For this review, take the finished solid that the model builds, in its own axes (mm). Face numbers are marked on the shaded views. A direction names the side the tool comes from. Give positions to 0.01 mm unless a question says otherwise; leave off trailing zeros. Write each loop counter-clockwise with the first axis right and the second up, starting at its lowest first coordinate (ties: lowest second). Pieces come first, ordered by that corner, then holes. Notation, with made-up numbers: (9.5, 15.25) -> (19.5, 15.25) arc R30 cw to (19.5, 40.25) -> close; hole circle Ø7 at (25.5, 88.25). An arc over 180 degrees is marked (long way). Return JSON: item names as keys, results as strings.
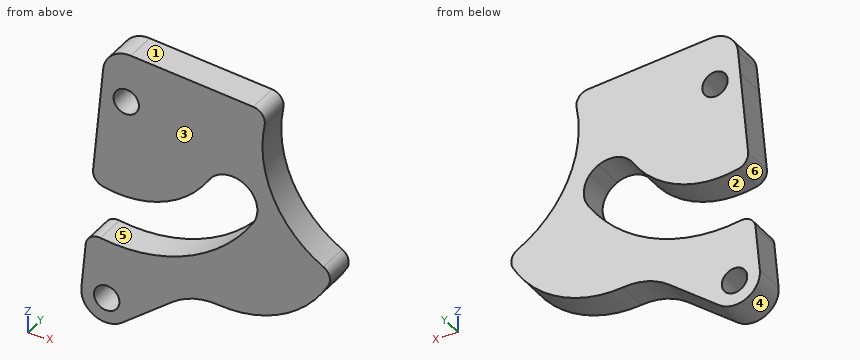
from build123d import *

# Parameters (mm, degrees)
SKETCH_1_R          = 2
EXTRUDE_1_DEPTH     = 5
EXTRUDE_2_DEPTH     = 5
CUT_EXTRUDE_1_DEPTH = 6
EXTRUDE_3_DEPTH     = 5
FILLET_1_R          = 10
FILLET_2_R          = 2
SKETCH_6_R          = 18.75
CUT_EXTRUDE_2_DEPTH = 6
FILLET_3_R          = 2


with BuildPart() as part:
    # 草图1 → 凸台-拉伸1 (new body)
    with BuildSketch(Plane(origin=(0, 0, 0), x_dir=(1, 0, 0), z_dir=(0, 1, 0))):
        with BuildLine():
            ThreePointArc((-20.0875, 4), (-23.044826598, 2.693365811), (-24.070081176, -0.372890305))
            ThreePointArc((-24.070081176, -0.372890305), (-22.780865811, -2.957326598), (-20.0875, -4))
            ThreePointArc((-20.0875, -4), (-17.130173402, -2.693365811), (-16.104918824, 0.372890305))
            Line((-16.104918824, 0.372890305), (-16.444526225, 4))
            Line((-16.444526225, 4), (-20.0875, 4))
        make_face()
        with Locations((-20.0875, 0)):
            Circle(SKETCH_1_R, mode=Mode.SUBTRACT)
        with BuildLine():
            Line((-27.14754486, 32.495352138), (-24.070081176, -0.372890305))
            ThreePointArc((-24.070081176, -0.372890305), (-23.044826598, 2.693365811), (-20.0875, 4))
            Line((-20.0875, 4), (-16.444526225, 4))
            Line((-16.444526225, 4), (-18.333300994, 24.172685504))
            Line((-18.333300994, 24.172685504), (-25.585127327, 29.683464909))
            ThreePointArc((-25.585127327, 29.683464909), (-26.661456606, 30.925425609), (-27.14754486, 32.495352138))
        make_face()
        with BuildLine():
            ThreePointArc((-20.74480004, 36.053019976), (-25.107780517, 36.364735365), (-27.14754486, 32.495352138))
            ThreePointArc((-27.14754486, 32.495352138), (-26.661456606, 30.925425609), (-25.585127327, 29.683464909))
            Line((-25.585127327, 29.683464909), (-18.333300994, 24.172685504))
            Line((-18.333300994, 24.172685504), (-19.182382508, 33.241132747))
            ThreePointArc((-19.182382508, 33.241132747), (-19.668470762, 34.811059276), (-20.74480004, 36.053019976))
        make_face()
        with Locations((-23.164963684, 32.868242443)):
            Circle(SKETCH_1_R, mode=Mode.SUBTRACT)
        with BuildLine():
            Line((22.507663644, 3.184777534), (-20.74480004, 36.053019976))
            ThreePointArc((-20.74480004, 36.053019976), (-19.668470762, 34.811059276), (-19.182382508, 33.241132747))
            Line((-19.182382508, 33.241132747), (-18.333300994, 24.172685504))
            Line((-18.333300994, 24.172685504), (8.212637649, 4))
            Line((8.212637649, 4), (20.0875, 4))
            ThreePointArc((20.0875, 4), (21.364388771, 3.790719598), (22.507663644, 3.184777534))
        make_face()
        with BuildLine():
            ThreePointArc((-16.104918824, 0.372890305), (-17.130173402, -2.693365811), (-20.0875, -4))
            Line((-20.0875, -4), (20.0875, -4))
            ThreePointArc((20.0875, -4), (18.810611229, -3.790719598), (17.667336356, -3.184777534))
            Line((17.667336356, -3.184777534), (8.212637649, 4))
            Line((8.212637649, 4), (-16.444526225, 4))
            Line((-16.444526225, 4), (-16.104918824, 0.372890305))
        make_face()
        with BuildLine():
            ThreePointArc((17.667336356, -3.184777534), (18.810611229, -3.790719598), (20.0875, -4))
            ThreePointArc((20.0875, -4), (23.878219598, -1.276888771), (22.507663644, 3.184777534))
            ThreePointArc((22.507663644, 3.184777534), (21.364388771, 3.790719598), (20.0875, 4))
            Line((20.0875, 4), (8.212637649, 4))
            Line((8.212637649, 4), (17.667336356, -3.184777534))
        make_face()
        with Locations((20.0875, 0)):
            Circle(SKETCH_1_R, mode=Mode.SUBTRACT)
        Polygon((-18.333300994, 24.172685504), (-16.444526225, 4), (8.212637649, 4), align=None)
    extrude(amount=EXTRUDE_1_DEPTH)

    # 草图2 → 凸台-拉伸2 (add)
    with BuildSketch(Plane(origin=(0, 5, 0), x_dir=(1, 0, 0), z_dir=(0, 1, 0))):
        with BuildLine():
            ThreePointArc((-20.0875, -4), (-22.780865811, -2.957326598), (-24.070081176, -0.372890305))
            Line((-24.070081176, -0.372890305), (-23.720962628, -4.10158193))
            ThreePointArc((-23.720962628, -4.10158193), (-22.290826699, -6.808468121), (-19.365512753, -7.711274824))
            Line((-19.365512753, -7.711274824), (20.460368699, -3.982583199))
            ThreePointArc((20.460368699, -3.982583199), (20.274137625, -3.995643427), (20.0875, -4))
            Line((20.0875, -4), (-20.0875, -4))
        make_face()
    extrude(amount=-EXTRUDE_2_DEPTH)

    # 草图3 → 切除-拉伸1 (cut, through all)
    with BuildSketch(Plane(origin=(0, 5, 0), x_dir=(1, 0, 0), z_dir=(0, 1, 0))):
        with BuildLine():
            ThreePointArc((-36.289327432, 17.433897667), (-37.629570165, 14.285674695), (-36.182704661, 11.185007239))
            ThreePointArc((-36.182704661, 11.185007239), (-31.653466249, 15.823666602), (-25.858788976, 18.731049718))
            Line((-25.858788976, 18.731049718), (-26.257218708, 22.986399698))
            ThreePointArc((-26.257218708, 22.986399698), (-31.612650276, 20.82332613), (-36.289327432, 17.433897667))
        make_face()
        with BuildLine():
            ThreePointArc((-25.858788976, 18.731049718), (-11.47348363, 17.605644606), (-1.756724615, 6.938492183))
            ThreePointArc((-1.756724615, 6.938492183), (0.40025314, 9.594618202), (-0.134776474, 12.974159854))
            ThreePointArc((-0.134776474, 12.974159854), (-11.569633945, 22.223545124), (-26.257218708, 22.986399698))
            Line((-26.257218708, 22.986399698), (-25.858788976, 18.731049718))
        make_face()
        with BuildLine():
            ThreePointArc((-7.176914189, 8.395044611), (-4.745829362, 6.62850376), (-1.756724615, 6.938492183))
            ThreePointArc((-1.756724615, 6.938492183), (-11.47348363, 17.605644606), (-25.858788976, 18.731049718))
            Line((-25.858788976, 18.731049718), (-25.456435977, 14.433798061))
            ThreePointArc((-25.456435977, 14.433798061), (-15.256790284, 14.622730376), (-7.176914189, 8.395044611))
        make_face()
        with BuildLine():
            ThreePointArc((-25.858788976, 18.731049718), (-31.653466249, 15.823666602), (-36.182704661, 11.185007239))
            ThreePointArc((-36.182704661, 11.185007239), (-33.358528619, 10.15793874), (-30.571035397, 11.280757314))
            ThreePointArc((-30.571035397, 11.280757314), (-28.168999159, 13.109133127), (-25.456435977, 14.433798061))
            Line((-25.456435977, 14.433798061), (-25.858788976, 18.731049718))
        make_face()
    extrude(amount=-CUT_EXTRUDE_1_DEPTH, mode=Mode.SUBTRACT)

    # 草图4 → 凸台-拉伸3 (add)
    with BuildSketch(Plane(origin=(0, 5, 0), x_dir=(1, 0, 0), z_dir=(0, 1, 0))):
        with BuildLine():
            ThreePointArc((13.821061528, 9.785866119), (13.838380431, 10.235085855), (13.844154668, 10.684602232))
            ThreePointArc((13.844154668, 10.684602232), (6.570974544, 24.885382325), (-9.202948787, 27.282181672))
            Line((-9.202948787, 27.282181672), (13.821061528, 9.785866119))
        make_face()
    extrude(amount=-EXTRUDE_3_DEPTH)

    # 圆角1
    fillet_1_edges = [part.edges().sort_by_distance(p)[0] for p in [
        (13.821061528, 2.5, -9.785866119),
        (-9.202948787, 2.5, -27.282181672),
    ]]
    fillet(fillet_1_edges, radius=FILLET_1_R)

    # 圆角2
    fillet_2_edges = [part.edges().sort_by_distance(p)[0] for p in [
        (-26.257218708, 2.5, -22.986399698),
        (-25.456435977, 2.5, -14.433798061),
    ]]
    fillet(fillet_2_edges, radius=FILLET_2_R)

    # 草图6 → 切除-拉伸2 (cut, through all)
    with BuildSketch(Plane(origin=(0, 5, 0), x_dir=(1, 0, 0), z_dir=(0, 1, 0))):
        with Locations((20.0875, 0)):
            Circle(SKETCH_6_R)
    extrude(amount=-CUT_EXTRUDE_2_DEPTH, mode=Mode.SUBTRACT)

    # 圆角3
    fillet_3_edges = [part.edges().sort_by_distance(p)[0] for p in [
        (12.591508983, 2.5, -17.186407963),
        (2.22176543, 2.5, 5.690169441),
    ]]
    fillet(fillet_3_edges, radius=FILLET_3_R)


solid = part.part
1. For the marked faces 5 and 6, list the 3-axis set-ups (+Z, -Z, +X, -X, +Y, -Y) from which the entire face can be reached by the end or side of a thin tool; tool diameter is ignored.
Results found:
{"face 5": "+Y, -Y", "face 6": "-X, +Y, -Y"}
2. Add section A-A, the plane x = -8. State the section outline as (y, z) points.
Results found:
{"outline": "(0, -28.08) -> (5, -28.08) -> (5, -20.5) -> (0, -20.5) -> close; (0, -9.54) -> (5, -9.54) -> (5, 6.65) -> (0, 6.65) -> close"}
3. Add section B-B, the plane y = 0.8. Count the separate pieces of the cut face and the enclosed holes in it, plus the area to 3 significant figures.
Results found:
{"separate pieces": "1", "enclosed holes": "2", "area": "878 mm²"}
4. For pin 1 (2 mm diameter, centred on y = 1, z = 3, fed in from +X); pin 2 (3 mm diameter, centred on x = 5, y = 3.5, fed in from -Z), all flat-tipped, find the tip position at first contact; note any pin that passes through.
Results found:
{"pin 1": "stops at x = 1.71", "pin 2": "stops at z = -26.65"}
5. The part is to be moulded in two halves that separate along X. For the marked faces 1, 2, 3 and 4, say which applies: +X half, -X half, draft (parallel to the pull), parting line (faces both ways), or undercut.
Results found:
{"face 1": "+X half", "face 2": "undercut", "face 3": "draft", "face 4": "parting line"}
6. To check wall thickness, follow probe 1 along Z at (x, y) = (-18, 1.4); probe 2 along Z at (x, y) = (-14, 4.25); probe 3 along X at (y, z) = (2.1, 0) (1 decimal). State the ranges of each line that lie inside material, in increasing order.
Results found:
{"probe 1": "z = -33.97 to -23.71, -15.26 to 7.58", "probe 2": "z = -30.93 to -23.01, -14.15 to 7.21", "probe 3": "x = -24.1 to -22.1, -18.1 to 1.3"}
